Source: CAD feature listing. Evaluate the final solid. Frame: model axes, mm. A direction names the side the tool comes from. Coordinates: 2 decimals unless noted, no trailing zeros. Order: outer loops, then holes, each group sorted by start corner. A loop starts at its lowest first (then second) coordinate and runs counter-clockwise, first axis right, second up.
```python
from build123d import *

# Parameters (mm, degrees)
SKETCH1_R               = 6.35
SKETCH1_W               = 15
SKETCH1_H               = 20.4
SKETCH1_R_2             = 1.5
BOSS_EXTRUDE1_DEPTH     = 40
CUT_EXTRUDE1_START      = -3.5
SKETCH1_7_W             = 15
SKETCH1_7_H             = 20.4
SKETCH1_7_R             = 1.5
CUT_EXTRUDE1_DEPTH      = 4.5
CUT_EXTRUDE2_START      = -10
CUT_EXTRUDE2_DEPTH      = 20
FILLET1_R               = 5
CUT_EXTRUDE3_DEPTH      = 39.804456485
CUT_EXTRUDE3_DEPTH_BACK = 39.804456485
CHAMFER1_SIZE           = 28
CHAMFER1_SIZE_2         = 11.885294854
CUT_EXTRUDE5_DEPTH      = 46.945211938
CUT_EXTRUDE5_DEPTH_BACK = 20
SKETCH5_R               = 2.5


with BuildPart() as part:
    # Sketch1 → Boss-Extrude1 (new body)
    # profile 1 of 2: a face of its own
    with BuildSketch(Plane.XY):
        Polygon((-20.773681501, -13.2), (-15, -13.2), (15, -13.2), (15, -10.2), (0, -10.2), (0, 10.2), (15, 10.2), (15, 13.2), (-14.707827622, 13.2), (-15, 13.2), (-20.773681501, 13.2), align=None)
        with Locations((-10, 0)):
            Circle(SKETCH1_R, mode=Mode.SUBTRACT)
    # profile 2 of 2: a face of its own
    with BuildSketch(Plane.XY):
        with Locations((7.5, 0)):
            Rectangle(SKETCH1_W, SKETCH1_H)
        with Locations((4, -6.2)):
            Circle(SKETCH1_R_2, mode=Mode.SUBTRACT)
        with Locations((4, 6.2)):
            Circle(SKETCH1_R_2, mode=Mode.SUBTRACT)
    extrude(amount=-BOSS_EXTRUDE1_DEPTH)

    # Sketch1<7> → Cut-Extrude1 (cut)
    with BuildSketch(Plane.XY.offset(CUT_EXTRUDE1_START)):
        with Locations((7.5, 0)):
            Rectangle(SKETCH1_7_W, SKETCH1_7_H)
        with Locations((4, -6.2)):
            Circle(SKETCH1_7_R, mode=Mode.SUBTRACT)
        with Locations((4, 6.2)):
            Circle(SKETCH1_7_R, mode=Mode.SUBTRACT)
    extrude(amount=-CUT_EXTRUDE1_DEPTH, mode=Mode.SUBTRACT)

    # Sketch2 → Cut-Extrude2 (cut)
    with BuildSketch(Plane.XY.offset(CUT_EXTRUDE2_START)):
        with BuildLine():
            Line((-0.235583945, 2.157818136), (-2.675772908, 13.2))
            Line((-2.675772908, 13.2), (-11.927619652, 13.2))
            Line((-11.927619652, 13.2), (-20.773681501, 13.2))
            Line((-20.773681501, 13.2), (-20.773681501, -13.2))
            Line((-20.773681501, -13.2), (-2.675772908, -13.2))
            Line((-2.675772908, -13.2), (-0.235583945, -2.157818136))
            ThreePointArc((-0.235583945, -2.157818136), (0, 0), (-0.235583945, 2.157818136))
        make_face()
    extrude(amount=-CUT_EXTRUDE2_DEPTH, mode=Mode.SUBTRACT)

    # Fillet1
    fillet1_edges = [part.edges().sort_by_distance(p)[0] for p in [
        (-2.675772908, 13.2, -20),
        (-2.675772908, -13.2, -20),
    ]]
    fillet(fillet1_edges, radius=FILLET1_R)

    # Sketch3 → Cut-Extrude3 (cut, two sides: drawn at the far end of the back side and taken through both)
    with BuildSketch(Plane.XY.offset(-30).offset(-CUT_EXTRUDE3_DEPTH_BACK)):
        with BuildLine():
            Line((-10, 8.35), (1.266113946, 12.648007971))
            ThreePointArc((1.266113946, 12.648007971), (2.375075148, 13.060043202), (3.549800678, 13.2))
            Line((3.549800678, 13.2), (-20.773681501, 13.2))
            Line((-20.773681501, 13.2), (-20.773681501, -13.2))
            Line((-20.773681501, -13.2), (3.549800678, -13.2))
            ThreePointArc((3.549800678, -13.2), (2.375075148, -13.060043202), (1.266113946, -12.648007971))
            Line((1.266113946, -12.648007971), (-10, -8.35))
            ThreePointArc((-10, -8.35), (-18.35, 0), (-10, 8.35))
        make_face()
    extrude(amount=CUT_EXTRUDE3_DEPTH + CUT_EXTRUDE3_DEPTH_BACK, mode=Mode.SUBTRACT)

    # Chamfer1
    # the kernel refuses this chamfer: 28, 11.885294854 mm, written as the material it takes off along each edge
    with BuildSketch(Plane(origin=(15, 85.785659069, -40), x_dir=(0.01507249742986372, 0, 0.9998864034585262), z_dir=(0, -1, 0))) as chamfer1_piece_1:
        Polygon((CHAMFER1_SIZE * 0.999886403459, CHAMFER1_SIZE * 0.0150724974299), (-CHAMFER1_SIZE_2 * 0.0150724974297, CHAMFER1_SIZE_2 * 0.999886403448), (0, 0), align=None)
    extrude(amount=171.571318139, mode=Mode.SUBTRACT)

    # Sketch5 → Cut-Extrude5 (cut, two sides: drawn at the far end of the back side and taken through both)
    with BuildSketch(Plane(origin=(0, 0, -40), x_dir=(-1, 0, 0), z_dir=(0, 0, -1)).offset(-CUT_EXTRUDE5_DEPTH_BACK)):
        with Locations(Location((-4, 6.2, 0), (0, 0, 290.739394744))):
            Circle(SKETCH5_R)
        with Locations(Location((-4, -6.2, 0), (0, 0, 290.739394744))):
            Circle(SKETCH5_R)
    extrude(amount=CUT_EXTRUDE5_DEPTH + CUT_EXTRUDE5_DEPTH_BACK, mode=Mode.SUBTRACT)


solid = part.part
```
Q1. Set-up query: faces 1 (the flat face through (-0.79, -4.67, -19.86)), 2 (the cylindrical face through (1.553, 5.69, -27.638)), 3 (the flat face through (7, 0, -3.5)). Return all of +Z, -Z, +X, -X, +Y, -Y with unobstructed straight access to the full face (end or side cutting, diameter ignored); none if empty.
Solutions:
face 1: -X
face 2: -Z
face 3: +X
Q2. Section query B-B on z = -9.5. Output: boundary loops of the cut face in (x, y), plus the area to 3 significant figures.
Solutions:
outline: (-10, -8.35) - (1.27, -12.65) arc R5 ccw to (3.55, -13.2) - (15, -13.2) - (15, 13.2) - (3.55, 13.2) arc R5 ccw to (1.27, 12.65) - (-10, 8.35) arc R8.35 ccw to start; hole circle Ø12.7 at (-10, 0); hole circle Ø3 at (4, -6.2); hole circle Ø3 at (4, 6.2)
area: 567 mm2
Q3. Section query C-C on z = -4. Output: boundary loops of the cut face in (x, y), plus the area to 3 significant figures.
Solutions:
outline: (-10, -8.35) - (1.27, -12.65) arc R5 ccw to (3.55, -13.2) - (15, -13.2) - (15, -10.2) - (0, -10.2) - (0, 10.2) - (15, 10.2) - (15, 13.2) - (3.55, 13.2) arc R5 ccw to (1.27, 12.65) - (-10, 8.35) arc R8.35 ccw to start; hole circle Ø12.7 at (-10, 0)
area: 275 mm2
Q4. Section query D-D on x = -7.5. Output: boundary loops of the cut face in (y, z), plus the area to 3 significant figures.
Solutions:
outline: (-9.3, -40) - (-5.84, -40) - (-5.84, -30) - (-9.3, -30) - close; (-9.3, -10) - (-5.84, -10) - (-5.84, 0) - (-9.3, 0) - close; (5.84, -40) - (9.3, -40) - (9.3, -30) - (5.84, -30) - close; (5.84, -10) - (9.3, -10) - (9.3, 0) - (5.84, 0) - close
area: 139 mm2
Q5. Pull-direction query (Z, two-part tool) for faces 4 (the flat face through (-4.29, -10.53, -35.07)), 5 (the cylindrical face through (0, 0, -20)); classes: pulls with the +Z half, pulls with the -Z half, needs draft (parallel to the pull), parting line crosses it, or undercut.
Solutions:
face 4: needs draft
face 5: undercut
Q6. Pin query (flat end, axial travel): P1, Ø2, axis at y = -1.5, z = -33.5, coming from the -X side (3 decimals); P2, Ø1, axis at x = 11, y = -6.5, coming from the -Z side; P3, Ø4, axis at y = 8.5, z = -18.5, coming from the +X side; P4, Ø1.8, axis at x = 4, y = -6.2, coming from the -Z side. Return the tip coordinate at first contact, or that it passes through.
Solutions:
P1: stops at x = -18.335
P2: stops at z = -22.6
P3: stops at x = 13.09
P4: passes through
Q7. Material intervals for line 1 along Y through (x, z) = (4, -34); line 2 along Y through (x, z) = (4, -14); line 3 along Z through (x, y) = (-7.5, -6.75), sorted ascending.
Solutions:
line 1: y = -13.2 to -8.7, -3.7 to 3.7, 8.7 to 13.2
line 2: y = -13.2 to -7.7, -4.7 to 4.7, 7.7 to 13.2
line 3: z = -40 to -30, -10 to 0
Q8. Section query A-A on y = 0. Output: boundary loops of the cut face in (x, z).
Solutions:
outline: (-18.35, -40) - (-16.35, -40) - (-16.35, -30) - (-18.35, -30) - close; (-18.35, -10) - (-16.35, -10) - (-16.35, 0) - (-18.35, 0) - close; (-3.65, -40) - (3.11, -40) - (15, -12) - (15, -8) - (0, -8) - (0, -3.5) - (15, -3.5) - (15, 0) - (-3.65, 0) - (-3.65, -10) - (0, -10) - (0, -30) - (-3.65, -30) - close
